Geometry: final body of the model. Coordinates: model frame, mm. A direction names the side the tool comes from. Give positions to 0.01 mm unless a question says otherwise; leave off trailing zeros. Write each loop counter-clockwise with the first axis right and the second up, starting at its lowest first coordinate (ties: lowest second). Pieces come first, ordered by that corner, then holes. Notation, with made-up numbers: M 71.25,-2.5 L 86.25,-2.5 A10 ccw 86.25,12.5 Z; hole C 74,53 d6. An arc over 180 degrees is marked long. Use a Markdown table: item, result. Add a question column.
(1) Pin query (flat end, axial travel): pin 1 Ø8 at (x, z) = (3, 77) entering from +Y; pin 2 Ø3 at (y, z) = (-6.5, 62) entering from -X; pin 3 Ø15 at (x, y) = (7, 2) entering from -Z; pin 4 Ø6 at (x, y) = (13.5, 12) entering from +Z. Return the tip coordinate at first contact, or that it passes through.
(2) Reachability of faces 1 (the flat face through (12.86, 7.72, 95.45)), 2 (the flat face through (7.5, 7, 90)) from +Z, -Z, +X, -X, +Y, -Y: full face, straight path, thin tool, end or side. Return the list, or none.
(3) Draft query along Z for faces 3 (the flat face through (0, 0, 102.5)), 4 (the flat face through (-13.117, 7.278, 95.451)), 5 (the flat face through (0, 0, 0)). Return one class per face: released by +Z, released by -Z, zero draft, split by the parting line, or undercut.
(4) Cut plane A-A (z = 76). Output: boundary loops of the cut face in (x, y), plus the area to 3 significant figures.
(5) Cut plane B-B (x = 0). Output: boundary loops of the cut face in (y, z).
(6) Material intervals for L1, parallel to Z at x = -5, y = -10.5; L2, parallel to X at y = -2.5, z = 18; L3, parallel to X at y = -4, z = 69, sorted ascending.
```python
from build123d import *

# Parameters (mm, degrees)
SKETCH1_R           = 10
BOSS_EXTRUDE1_DEPTH = 90
BOSS_EXTRUDE2_DEPTH = 12.5
SKETCH4_OUTSIDE_W   = 76.428
SKETCH4_OUTSIDE_H   = 72.224
SKETCH4_OUTSIDE_R   = 12.5
CUT_EXTRUDE2_DEPTH  = 5
CUT_EXTRUDE2_DRAFT  = -60


with BuildPart() as part:
    # Sketch1 → Boss-Extrude1 (new body)
    with BuildSketch(Plane.XY):
        with Locations(Location((0, 0, 0), (0, 0, 180))):
            Circle(SKETCH1_R)
    extrude(amount=BOSS_EXTRUDE1_DEPTH)

    # Sketch3 → Boss-Extrude2 (add)
    with BuildSketch(Plane.XY.offset(90)):
        Polygon((8.280492797, 15.212936569), (-9.034543136, 14.777585402), (-17.315035933, -0.435351166), (-8.280492797, -15.212936569), (9.034543136, -14.777585402), (17.315035933, 0.435351166), align=None)
    extrude(amount=BOSS_EXTRUDE2_DEPTH)


with BuildPart() as cut_extrude2_tool:
    # Sketch4 outside → Cut-Extrude2 (with draft: the straight prism first)
    with BuildSketch(Plane.XY.offset(102.5)):
        Rectangle(SKETCH4_OUTSIDE_W, SKETCH4_OUTSIDE_H)
        Circle(SKETCH4_OUTSIDE_R, mode=Mode.SUBTRACT)
    extrude(amount=-CUT_EXTRUDE2_DEPTH)
    # Cut-Extrude2: the draft: its side faces are tilted about the plane it starts from
    cut_extrude2_sides = [cut_extrude2_tool.faces().sort_by_distance(p)[0] for p in [
        (0, -36.112, 100),
        (38.214, 0, 100),
        (0, 36.112, 100),
        (-38.214, 0, 100),
        (-12.5, 0, 100),
    ]]
    draft(cut_extrude2_sides, Plane.XY.offset(102.5), CUT_EXTRUDE2_DRAFT)


with BuildPart() as part_1:
    add(part.part)

    # Cut-Extrude2: cut by cut_extrude2_tool
    add(cut_extrude2_tool.part, mode=Mode.SUBTRACT)


solid = part_1.part
```
Answer list:
| question | item | result |
|---|---|---|
| 1 | pin 1 | y = 10 |
| 1 | pin 2 | x = -8.66 |
| 1 | pin 3 | z = 0 |
| 1 | pin 4 | z = 101.02 |
| 2 | face 1 | +Z, -Z, +X, +Y |
| 2 | face 2 | -Z |
| 3 | face 3 | released by +Z |
| 3 | face 4 | zero draft |
| 3 | face 5 | released by -Z |
| 4 | outline | C 0,0 d20 |
| 4 | area | 314 mm² |
| 5 | outline | M -15,90 L -10,90 L -10,0 L 10,0 L 10,90 L 15,90 L 15,101.05 L 12.5,102.5 L -12.5,102.5 L -15,101.05 Z |
| 6 | L1 | 90 to 102.5 |
| 6 | L2 | -9.68 to 9.68 |
| 6 | L3 | -9.17 to 9.17 |
